Autodesk Fusion 360 part; units mm, degrees
sketch "Sketch1" plane through (0, 0, 0) normal (0, 1, 0) x (1, 0, 0)
  circle A0 centre (0, 0) radius 50
  dimension "d1" = 100
extrude "Extrude1" add sketch "Sketch1" along normal blind 200
hole "Hole1" at (-0.8268, 0, 0.2116) direction (0, 1, 0) diameter 90 depth 190 tip angle 180 countersink diameter 95 countersink angle 90
sketch "Sketch2" plane through (0, 0, 0) normal (0, 0, 1) x (1, 0, 0)
  circle A0 centre (-40, 185) radius 5
  dimension "d9" = 10
extrude "Extrude2" cut sketch "Sketch2" along normal blind 60
hole "Hole2" at (-0.2581, 190, -0.086) direction (0, 1, 0) diameter 10 depth 4411.663 tip angle 180 countersink diameter 80 countersink angle 175
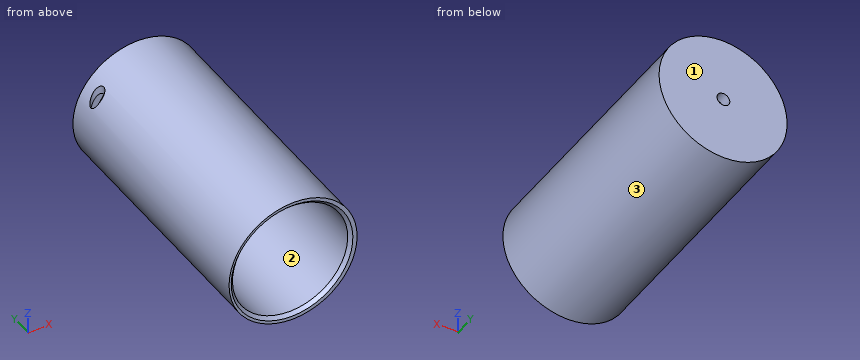
Here's how the part is built. I have some questions about the finished solid (model axes, mm). Face numbers are marked on the shaded views. Coordinates: 2 decimals unless noted, no trailing zeros. Loops run counter-clockwise (first coordinate to the right, second up) from the corner with the lowest first, then second, coordinate; pieces in that order, holes last. Notation, with made-up numbers: M 75,-27.75 L 119,-27.75 A20 ccw 119,-15.75 Z; hole C -4,7.25 d10. An arc over 180 degrees is marked long. One line per item, written item: value.
1. Thinking about a two-plate mould opening in Z: for the marked faces 1, 2 and 3, which applies, +Z half, -Z half, draft (parallel to the pull), parting line (faces both ways), or undercut?
Geometry says:
face 1: draft
face 2: undercut
face 3: parting line
2. Imagine slicing it at B-B (y = 185). List the corners of the cut face in (x, z) for me, and give its area (3 significant figures).
Geometry says:
outline: M -45,8.8 L -45,21.79 A50 ccw long -35,35.71 L -35,29.49 A45 cw long Z
area: 1,410 mm2
3. Will these pins go through, and if not, where does the flat tip stop? pin 1 Ø1 at (y, z) = (71.5, 26) entering from +X; pin 2 Ø4 at (y, z) = (93, -16) entering from -X; pin 3 Ø3 at (x, z) = (-23.5, 22) entering from -Y.
Geometry says:
pin 1: stops at x = 43.01
pin 2: stops at x = -48
pin 3: stops at y = 190.28
4. Please list where these lines run through material, in increasing order: probe 1 along X at (y, z) = (36, -1.5); probe 2 along Y at (x, z) = (26, -29.5); probe 3 along Z at (x, y) = (-21.5, 107).
Geometry says:
probe 1: x = -49.98 to -45.79, 44.14 to 49.98
probe 2: y = 190.02 to 200
probe 3: z = -45.14 to -39.76, 40.18 to 45.14
5. Imagine slicing it at A-A (y = 64.5). List the corners of the cut face in (x, z) for me, and give its area (3 significant figures).
Geometry says:
outline: C 0,0 d100; hole C -0.83,0.21 d90
area: 1,490 mm2
